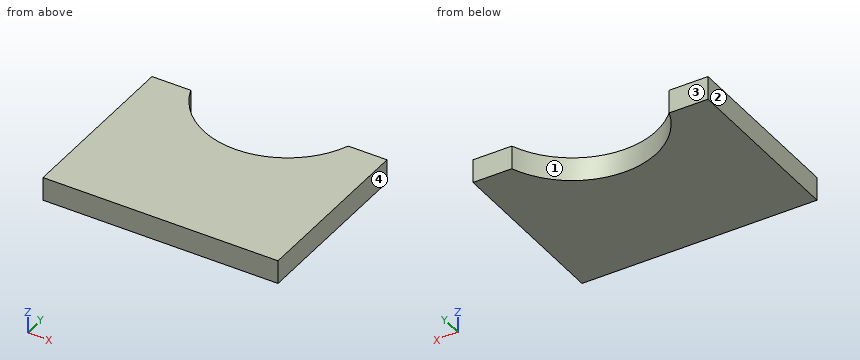
```python
from build123d import *

# Parameters (mm, degrees)
SKETCH1_W           = 40
SKETCH1_H           = 30
BOSS_EXTRUDE1_DEPTH = 4
CUT_EXTRUDE3_REACH  = 39.417
SKETCH5_R           = 14.3


with BuildPart() as part:
    # Sketch1 → Boss-Extrude1 (new body)
    with BuildSketch(Plane.XY.offset(-47.75)):
        with Locations((-2, 15)):
            Rectangle(SKETCH1_W, SKETCH1_H)
    extrude(amount=BOSS_EXTRUDE1_DEPTH)

    # Sketch5 → Cut-Extrude3 (cut, up to next)
    with BuildSketch(Plane.XY.offset(-43.75), mode=Mode.PRIVATE) as cut_extrude3_sk1:
        with Locations((-2, 35)):
            Circle(SKETCH5_R)
    cut_extrude3_tool1 = extrude(cut_extrude3_sk1.sketch, amount=-CUT_EXTRUDE3_REACH, mode=Mode.PRIVATE) & part.part
    add(cut_extrude3_tool1.solids().sort_by_distance((-2, 35, -43.75))[0], mode=Mode.SUBTRACT)


solid = part.part
```
For this review, take the finished solid that the model builds, in its own axes (mm). Face numbers are marked on the shaded views. Round coordinates to 2 decimals unless told otherwise and drop trailing zeros. Write each loop counter-clockwise with the first axis right and the second up, starting at its lowest first coordinate (ties: lowest second). Pieces come first, ordered by that corner, then holes.
1) For line 1 along X through (y, z) = (26.5, -44.35); line 2 along Y through (x, z) = (10, -44.95); line 3 along Y through (x, z) = (4.5, -44.9), list the stretches that pass through material, from the lowest coordinate up.
Answer below:
line 1: x = -22 to -13.5, 9.5 to 18
line 2: y = 0 to 27.22
line 3: y = 0 to 22.26
2) Mouldability with a two-part tool opening along X and no side actions: class the marked faces 1, 2, 3 and 4 as +X half, -X half, draft (parallel to the pull), parting line (faces both ways), or undercut.
Answer below:
face 1: undercut
face 2: -X half
face 3: draft
face 4: +X half
3) Take a section at C-C on x = 4.5. Give the boundary of the cut face in (y, z).
Answer below:
outline: (0, -47.75) - (22.26, -47.75) - (22.26, -43.75) - (0, -43.75) - close
4) Take a section at D-D on x = -1.5. Give the boundary of the cut face in (y, z), then the cut area to 3 significant figures.
Answer below:
outline: (0, -47.75) - (20.71, -47.75) - (20.71, -43.75) - (0, -43.75) - close
area: 82.8 mm2
5) Take a section at B-B on z = -45.1. Give the boundary of the cut face in (x, y).
Answer below:
outline: (-22, 0) - (18, 0) - (18, 30) - (11.4, 30) arc R14.3 cw to (-15.4, 30) - (-22, 30) - close
6) Take a section at A-A on y = 27. Give the boundary of the cut face in (x, z).
Answer below:
outline: (-22, -47.75) - (-13.85, -47.75) - (-13.85, -43.75) - (-22, -43.75) - close; (9.85, -47.75) - (18, -47.75) - (18, -43.75) - (9.85, -43.75) - close
